```python
from build123d import *

# Parameters (mm, degrees)
F0_W     = 40
F0_H     = 50
F1_DEPTH = 10
F3_DEPTH = 10.001


with BuildPart() as f1:
    # F0 (on Front) → F1 (new body)
    with BuildSketch(Plane.XZ):
        with Locations((20, 25)):
            Rectangle(F0_W, F0_H)
    extrude(amount=F1_DEPTH)

    # F2 (on face) → F3 (cut, through all)
    with BuildSketch(Plane.XZ.offset(10)):
        with BuildLine():
            Line((3.017207, 12.76887), (2, 7))
            ThreePointArc((2, 7), (2.828279, 3.263877), (6.055798, 1.20772))
            Line((6.055798, 1.20772), (6.055798, 0))
            Line((6.055798, 0), (40, 0))
            Line((40, 0), (40, 50))
            Line((40, 50), (29.800625, 50))
            Line((29.800625, 50), (29.800625, 43.731))
            ThreePointArc((29.800625, 43.731), (26.064502, 42.902721), (24.008346, 39.675202))
            Line((24.008346, 39.675202), (22.991119, 33.906221))
            ThreePointArc((22.991119, 33.906221), (22.284063, 32.088005), (20.935041, 30.678757))
            Line((20.935041, 30.678757), (9.185442, 22.451263))
            ThreePointArc((9.185442, 22.451263), (5.138375, 18.22352), (3.017207, 12.76887))
        make_face()
    extrude(amount=-F3_DEPTH, mode=Mode.SUBTRACT)


solid = f1.part
```
Verification items for the finished model (mm, model axes). A direction names the side the tool comes from. Round coordinates to 2 decimals unless told otherwise and drop trailing zeros. Order: outer loops, then holes, each group sorted by start corner. A loop starts at its lowest first (then second) coordinate and runs counter-clockwise, first axis right, second up. Notation, with made-up numbers: (6, 26) - (36, 26) arc R30 cw to (36, 61) - close; hole circle Ø8 at (56, 54.25). An arc over 180 degrees is marked (long way). Use CSV: the item, a comma, the result in double quotes. Start each with the question number.
1) Section check D-D, the plane x = 27.5. Record the cut outline in (y, z), plus the area to 3 significant figures.
2) Mould release check, pull along Z, two halves, no side actions. Record for faces 3 (the flat face through (11, 0, 36)), 4 (the flat face through (2.516, -5.07, 9.925)), 5 (the cylindrical face through (5, -5, 18)), 6 (the flat face through (3, -5, 0)): +Z half, -Z half, draft (parallel to the pull), parting line (faces both ways), or undercut.
3) Section check B-B, the plane y = -7. Record the cut outline in (x, z), plus the area to 3 significant figures.
4) Go/stop test with flat-tipped pins: P1, Ø3, axis at y = -9, z = 7, coming from the -X side; P2, Ø5, axis at x = 13.5, z = 20, coming from the +Y side; P3, Ø1.3, axis at y = -7, z = 0.5, coming from the +X side. Record where each tip stops, or that it passes through.
5) Section check A-A, the plane x = 5.5. Record the cut outline in (y, z).
6) Section check C-C, the plane z = 35. Record the cut outline in (x, y).
7) Access from +Z, -Z, +X, -X, +Y, -Y to the whole of each face (thin tool, end or side, straight path). Record for faces 1 (the flat face through (6.056, -5, 1)), 2 (the flat face through (11, -10, 36)).
8) Thickness scan on L1, parallel to Z at x = 5.5, y = -9; L2, parallel to X at y = -3.25, z = 19.5; L3, parallel to Z at x = 27.5, y = -3.5. Record the ranges inside material, lowest first.
Answers:
1,outline,"(-10, 43.6) - (0, 43.6) - (0, 50) - (-10, 50) - close"
1,area,"64.0 mm²"
2,face 3,"draft"
2,face 4,"undercut"
2,face 5,"undercut"
2,face 6,"-Z half"
3,outline,"(0, 0) - (6.06, 0) - (6.06, 1.21) arc R5 cw to (2, 7) - (3.02, 12.77) arc R15 cw to (9.19, 22.45) - (20.94, 30.68) arc R5 ccw to (22.99, 33.91) - (24.01, 39.68) arc R5 cw to (29.8, 43.73) - (29.8, 50) - (0, 50) - close"
3,area,"708 mm²"
4,P1,"stops at x = 0"
4,P2,"passes through"
4,P3,"stops at x = 6.06"
5,outline,"(-10, 0) - (0, 0) - (0, 1.34) - (-10, 1.34) - close; (-10, 18.76) - (0, 18.76) - (0, 50) - (-10, 50) - close"
6,outline,"(0, -10) - (23.18, -10) - (23.18, 0) - (0, 0) - close"
7,face 1,"-Z, +X, +Y, -Y"
7,face 2,"+Z, -Z, +X, -X, -Y"
8,L1,"z = 0 to 1.34, 18.76 to 50"
8,L2,"x = 0 to 6.05"
8,L3,"z = 43.6 to 50"
